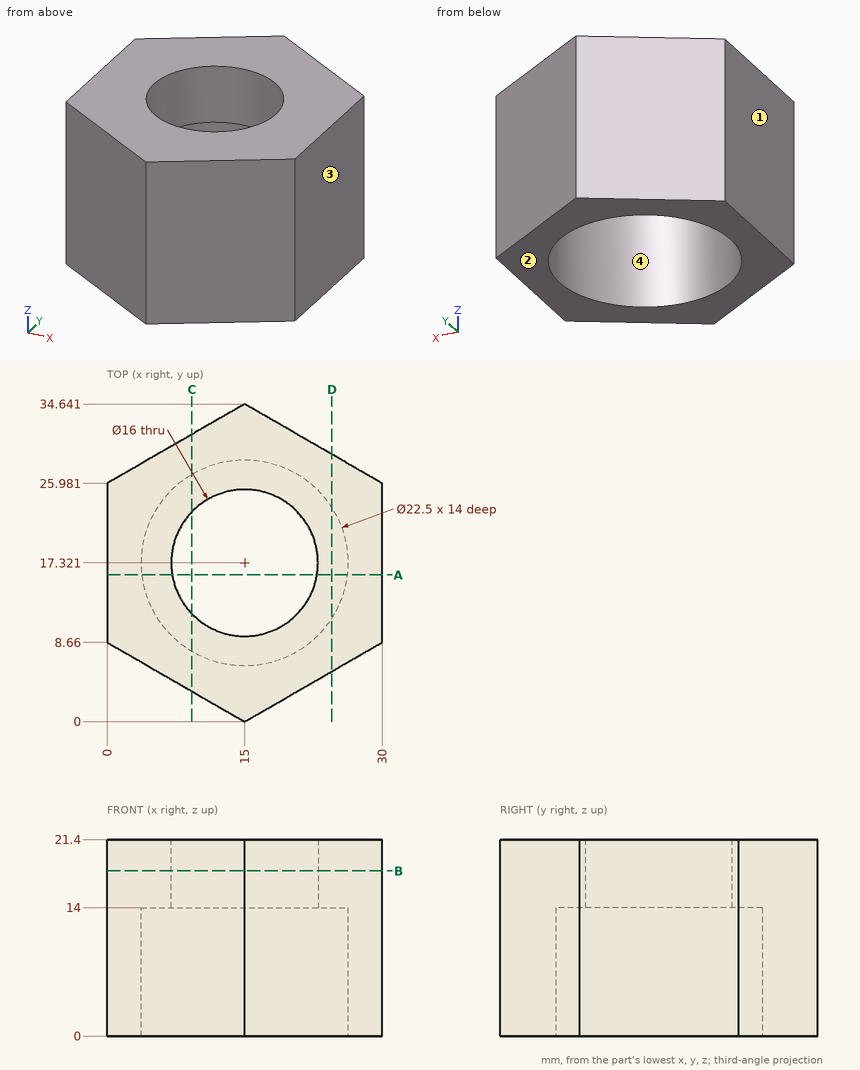
Part print with two shaded views. Sizes in mm from the minimum x, y, z corner. Round coordinates to 2 decimals unless told otherwise and drop trailing zeros. Order: outer loops, then holes, each group sorted by start corner. A loop starts at its lowest first (then second) coordinate and runs counter-clockwise, first axis right, second up. Notation, with made-up numbers: (17.25, -14.5) - (69.25, -14.5) arc R25 ccw to (69.25, 8.5) - close; hole circle Ø4 at (-2, 77.5). An arc over 180 degrees is marked (long way). Answer in a Markdown table with one row per item. Add a question column.
(1) Mould opens along X. For the marked faces 1, 2, 3 and 4 say: +X half, -X half, draft (parallel to the pull), parting line (faces both ways), or undercut.
(2) Band-saw the part on A-A on y = 16. List the corners of the cut face in (x, z).
(3) Band-saw the part on D-D on x = 24.5. List the corners of the cut face in (y, z) (1 decimal).
(4) Drop flat-ended pins along their axis: pin 1 Ø3 at (y, z) = (16.5, 6.5) entering from -X; pin 2 Ø1 at (x, z) = (20, 13) entering from +Y; pin 3 Ø1.5 at (x, z) = (6.5, 8.5) entering from -Y (1 decimal); pin 4 Ø2 at (x, y) = (26, 30) entering from -Z. Give the stop position or say it passes through.
(5) Band-saw the part on B-B on z = 18. List the corners of the cut face in (x, y).
(6) Band-saw the part on C-C on x = 9.25. List the corners of the cut face in (y, z), and give its area (3 significant figures).
(7) Probe L1, parallel to Y at x = 15, z = 6.75; L2, parallel to Y at x = 15, z = 16.5; L3, parallel to X at y = 21.5, z = 18.75. List the from-to ranges inside material, lowest first. Write a range as [from, to].
Data:
| question | item | result |
|---|---|---|
| 1 | face 1 | -X half |
| 1 | face 2 | draft |
| 1 | face 3 | +X half |
| 1 | face 4 | undercut |
| 2 | outline | (0, 0) - (3.83, 0) - (3.83, 14) - (7.11, 14) - (7.11, 21.4) - (0, 21.4) - close; (22.89, 14) - (26.17, 14) - (26.17, 0) - (30, 0) - (30, 21.4) - (22.89, 21.4) - close |
| 3 | outline | (5.5, 0) - (11.3, 0) - (11.3, 14) - (23.3, 14) - (23.3, 0) - (29.2, 0) - (29.2, 21.4) - (5.5, 21.4) - close |
| 4 | pin 1 | stops at x = 0 |
| 4 | pin 2 | stops at y = 32.04 |
| 4 | pin 3 | stops at y = 4.5 |
| 4 | pin 4 | passes through |
| 5 | outline | (0, 8.66) - (15, 0) - (30, 8.66) - (30, 25.98) - (15, 34.64) - (0, 25.98) - close; hole circle Ø16 at (15, 17.32) |
| 6 | outline | (3.32, 0) - (7.65, 0) - (7.65, 14) - (11.76, 14) - (11.76, 21.4) - (3.32, 21.4) - close; (22.88, 14) - (26.99, 14) - (26.99, 0) - (31.32, 0) - (31.32, 21.4) - (22.88, 21.4) - close |
| 6 | area | 246 mm^2 |
| 7 | L1 | y = [0, 6.07], [28.57, 34.64] |
| 7 | L2 | y = [0, 9.32], [25.32, 34.64] |
| 7 | L3 | x = [0, 8.18], [21.82, 30] |
